Design review of the part built by this model. Coordinates are the model's own, in mm. A direction names the side the tool comes from. Coordinates: 2 decimals unless noted, no trailing zeros. Write each loop counter-clockwise with the first axis right and the second up, starting at its lowest first coordinate (ties: lowest second). Pieces come first, ordered by that corner, then holes. Notation, with made-up numbers: (6, 72.5) -> (33, 72.5) arc R18 cw to (33, 85.5) -> close; hole circle Ø9 at (-12.75, 88.5). An arc over 180 degrees is marked (long way). One line per question, with ' | ' between items. Start each with the question number.
Q1. Wall thickness on probe 1 along X at (y, z) = (21, 1.9); probe 2 along Z at (x, y) = (-3.5, 11.75): over which ranges is each line inside the solid? List them lowest first.
Q2. Add section B-B on z = -0.05. State the section outline as (x, y) points, and give its area (3 significant figures).
Q3. For faces 1 (the flat face through (-5.701, 13, 1)), 2 (the flat face through (-7, 13, 2.5)), list the 3-axis set-ups (+Z, -Z, +X, -X, +Y, -Y) from which the entire face can be reached by the end or side of a thin tool; tool diameter is ignored.
Q4. For P1, Ø1, axis at x = -4.5, y = 6, coming from the +Z side; P2, Ø2.5, axis at y = 7, z = 1.5, coming from the +X side; P3, Ø3, axis at y = 18, z = 0.5, coming from the +X side, all flat-tipped, find the tip position at first contact; note any pin that passes through.
Q5. Add section A-A on y = 24. State the section outline as (x, z) points, and give its area (3 significant figures).
Q6. Add section C-C on x = -3.6. State the section outline as (y, z) points, and give its area (3 significant figures).
from build123d import *

# Parameters (mm, degrees)
BOSS_EXTRUDE1_DEPTH = 27


with BuildPart() as part:
    # Sketch1 → Boss-Extrude1 (new body)
    with BuildSketch(Plane(origin=(0, 0, 0), x_dir=(1, 0, 0), z_dir=(0, 1, 0))):
        Polygon((-6.432391634, 2.5), (-2.701042517, 2.5), (-2.701042517, 0.5), (-5.701042517, 0.5), (-5.701042517, -2.5), (-7.701042517, -2.5), (-7.701042517, 2.5), align=None)
    extrude(amount=BOSS_EXTRUDE1_DEPTH)


solid = part.part
Output values:
1) probe 1: x = -7.7 to -5.7 | probe 2: z = -2.5 to -0.5
2) outline: (-7.7, 0) -> (-5.7, 0) -> (-5.7, 27) -> (-7.7, 27) -> close | area: 54.0 mm2
3) face 1: +Z, +X, +Y, -Y | face 2: +Z, +X, -X, +Y, -Y
4) P1: stops at z = -0.5 | P2: stops at x = -5.7 | P3: stops at x = -2.7
5) outline: (-7.7, -2.5) -> (-2.7, -2.5) -> (-2.7, -0.5) -> (-5.7, -0.5) -> (-5.7, 2.5) -> (-7.7, 2.5) -> close | area: 16.0 mm2
6) outline: (0, -2.5) -> (27, -2.5) -> (27, -0.5) -> (0, -0.5) -> close | area: 54.0 mm2
